from build123d import *

# Parameters (mm, degrees)
SKETCH1_W           = 23
SKETCH1_H           = 32
BOSS_EXTRUDE1_DEPTH = 3.5
CUT_EXTRUDE1_DEPTH  = 1.075
FILLET1_R           = 6
FILLET2_R           = 5
FILLET3_R           = 2
CUT_EXTRUDE2_DEPTH  = 21.910523666
SKETCH5_R           = 6.9
CUT_EXTRUDE3_DEPTH  = 2.05


with BuildPart() as part:
    # Sketch1 → Boss-Extrude1 (new, symmetric)
    with BuildSketch(Plane.XY):
        Rectangle(SKETCH1_W, SKETCH1_H)
    extrude(amount=BOSS_EXTRUDE1_DEPTH, both=True)

    # Sketch2 → Cut-Extrude1 (cut, symmetric)
    with BuildSketch(Plane.XY):
        Polygon((-9.45, 16), (-11.5, 16), (-11.5, -16), (11.5, -16), (11.5, 16), (9.45, 16), (9.45, -13.95), (-9.45, -13.95), align=None)
    extrude(amount=CUT_EXTRUDE1_DEPTH, both=True, mode=Mode.SUBTRACT)

    # Fillet1
    fillet1_edges = [part.edges().sort_by_distance(p)[0] for p in [
        (-9.45, -13.95, 0),
        (9.45, -13.95, 0),
    ]]
    fillet(fillet1_edges, radius=FILLET1_R)

    # Fillet2
    fillet2_edges = [part.edges().sort_by_distance(p)[0] for p in [
        (11.5, -16, -2.2875),
        (-11.5, -16, -2.2875),
        (11.5, -16, 2.2875),
        (-11.5, -16, 2.2875),
    ]]
    fillet(fillet2_edges, radius=FILLET2_R)

    # Fillet3
    fillet3_edges = [part.edges().sort_by_distance(p)[0] for p in [
        (0, 16, 3.5),
        (-11.5, 2.5, 3.5),
        (0, 16, -3.5),
        (0, -16, -3.5),
        (11.5, 2.5, -3.5),
        (10.035533906, -14.535533906, -3.5),
        (-10.035533906, -14.535533906, -3.5),
        (-11.5, 2.5, -3.5),
        (0, -16, 3.5),
        (11.5, 2.5, 3.5),
        (10.035533906, -14.535533906, 3.5),
        (-10.035533906, -14.535533906, 3.5),
    ]]
    fillet(fillet3_edges, radius=FILLET3_R)

    # Sketch3 → Cut-Extrude2 (cut, through all)
    with BuildSketch(Plane.XY.offset(3.5)):
        with BuildLine():
            Line((-5.675, 3.418332927), (-5.675, -3.418332927))
            ThreePointArc((-5.675, -3.418332927), (0, -6.625), (5.675, -3.418332927))
            Line((5.675, -3.418332927), (5.675, 3.418332927))
            ThreePointArc((5.675, 3.418332927), (0, 6.625), (-5.675, 3.418332927))
        make_face()
    extrude(amount=-CUT_EXTRUDE2_DEPTH, mode=Mode.SUBTRACT)

    # Sketch5 → Cut-Extrude3 (cut)
    with BuildSketch(Plane.XY.offset(3.5)):
        Circle(SKETCH5_R)
    extrude(amount=-CUT_EXTRUDE3_DEPTH, mode=Mode.SUBTRACT)


solid = part.part
Verification items for the finished model (mm, model axes). A direction names the side the tool comes from. Coordinates: 2 decimals unless noted, no trailing zeros. Order: outer loops, then holes, each group sorted by start corner. A loop starts at its lowest first (then second) coordinate and runs counter-clockwise, first axis right, second up.
1. Sectioned sample at A-A, the plane y = 0. Record the cut outline in (x, z) (3 decimals), and give its area (3 significant figures).
Results found:
outline: (-11.5, -1.5) arc R2 ccw to (-9.5, -3.5) - (-5.675, -3.5) - (-5.675, 1.45) - (-6.9, 1.45) - (-6.9, 3.5) - (-9.5, 3.5) arc R2 ccw to (-11.5, 1.5) - (-11.5, 1.075) - (-9.45, 1.075) - (-9.45, -1.075) - (-11.5, -1.075) - close; (5.675, -3.5) - (9.5, -3.5) arc R2 ccw to (11.5, -1.5) - (11.5, -1.075) - (9.45, -1.075) - (9.45, 1.075) - (11.5, 1.075) - (11.5, 1.5) arc R2 ccw to (9.5, 3.5) - (6.9, 3.5) - (6.9, 1.45) - (5.675, 1.45) - close
area: 64.3 mm2
2. Sectioned sample at B-B, the plane x = 0. Record the cut outline in (y, z) (3 decimals).
Results found:
outline: (-16, -1.5) arc R2 ccw to (-14, -3.5) - (-6.625, -3.5) - (-6.625, 1.45) - (-6.9, 1.45) - (-6.9, 3.5) - (-14, 3.5) arc R2 ccw to (-16, 1.5) - (-16, 1.075) - (-13.95, 1.075) - (-13.95, -1.075) - (-16, -1.075) - close; (6.625, -3.5) - (14, -3.5) arc R2 ccw to (16, -1.5) - (16, 1.5) arc R2 ccw to (14, 3.5) - (6.9, 3.5) - (6.9, 1.45) - (6.625, 1.45) - close
3. Release check for a two-part mould opening along Y. For faces 1 (the face through (-10.93, 2.31, -2.9)), 2 (the face through (-0.095, -6.624, -0.99)), 3 (the face through (7.739, -12.146, -0.015)), 4 (the face through (6, 0, 1.45)) record: +Y half, -Y half, draft (parallel to the pull), parting line (faces both ways), or undercut.
Results found:
face 1: draft
face 2: undercut
face 3: -Y half
face 4: undercut
4. Go/stop test with flat-tipped pins: pin 1 Ø2 at (y, z) = (-1, 1) entering from -X; pin 2 Ø3 at (x, y) = (3.5, 0.5) entering from +Z; pin 3 Ø0.6 at (x, z) = (0.5, 0.5) entering from -Y; pin 4 Ø0.6 at (y, z) = (6, -0.5) entering from -X. Record where each tip stops, or that it passes through.
Results found:
pin 1: stops at x = -11.5
pin 2: passes through
pin 3: stops at y = -13.95
pin 4: stops at x = -9.45
5. Sectioned sample at D-D, the plane y = 12. Record the cut outline in (x, z) (3 decimals).
Results found:
outline: (-11.5, -1.5) arc R2 ccw to (-9.5, -3.5) - (9.5, -3.5) arc R2 ccw to (11.5, -1.5) - (11.5, -1.075) - (9.45, -1.075) - (9.45, 1.075) - (11.5, 1.075) - (11.5, 1.5) arc R2 ccw to (9.5, 3.5) - (-9.5, 3.5) arc R2 ccw to (-11.5, 1.5) - (-11.5, 1.075) - (-9.45, 1.075) - (-9.45, -1.075) - (-11.5, -1.075) - close
6. Set-up check for faces 5 (the face through (-9.45, 4, 0)), 6 (the face through (-7.646, -12.239, -0.015)), 7 (the face through (9.45, 4, 0)), 8 (the face through (0.095, 6.624, -0.99)), 9 (the face through (-0.1, -14.1, 1.075)): record each of +Z, -Z, +X, -X, +Y, -Y from which the full face is reachable in a straight line by a thin tool's end or side.
Results found:
face 5: -X, +Y, -Y
face 6: -X, -Y
face 7: +X, +Y, -Y
face 8: +Z, -Z
face 9: -Y
7. Scan lines: line 1 (X direction, y = 2, z = 1) (3 decimals); line 2 (Z direction, x = -9.5, y = -12) (3 decimals); line 3 (X direction, y = 14, z = 1). Record each from-to range of solid material in increasing order.
Results found:
line 1: x = -9.45 to -5.675, 5.675 to 9.45
line 2: z = -3.493 to -1.075, 1.075 to 3.493
line 3: x = -9.45 to 9.45
8. Sectioned sample at C-C, the plane z = 0.75. Record the cut outline in (x, y) (3 decimals).
Results found:
outline: (-9.45, -7.95) arc R6 ccw to (-3.45, -13.95) - (3.45, -13.95) arc R6 ccw to (9.45, -7.95) - (9.45, 16) - (-9.45, 16) - close; hole (-5.675, -3.418) arc R6.625 ccw to (5.675, -3.418) - (5.675, 3.418) arc R6.625 ccw to (-5.675, 3.418) - close
